from build123d import *
from build123d.topology import SkipClean

# Parameters (mm, degrees)
CUT_EXTRUDE1_DEPTH      = 35
CUT_EXTRUDE1_DEPTH_BACK = 35
SKETCH2_OUTSIDE_W       = 96.248
SKETCH2_OUTSIDE_H       = 96.248
BOSS_EXTRUDE1_DEPTH     = 46
SKETCH4_R               = 3.5
CUT_EXTRUDE2_DEPTH      = 5
LPATTERN1_COUNT         = 2
LPATTERN1_PITCH         = 35
SCALE1_SCALE            = 0.2286


with BuildPart() as part:
    # Sketch1 → Revolve2 (revolve)
    with BuildSketch(Plane(origin=(0, 0, 0), x_dir=(1, 0, 0), z_dir=(0, 1, 0))):
        with BuildLine():
            Line((0, 35), (0, -35))
            ThreePointArc((0, -35), (35, 0), (0, 35))
        make_face()
    revolve(axis=Axis((0, 0, -35), (0, 0, 1)))

    # Sketch2 outside → Cut-Extrude1 (cut, two sides: drawn at the far end of the back side and taken through both)
    with SkipClean():  # the faces are left unmerged after this step: merging them gives an invalid solid
        with BuildSketch(Plane(origin=(0, 0, 0), x_dir=(1, 0, 0), z_dir=(0, 1, 0)).offset(-CUT_EXTRUDE1_DEPTH_BACK)):
            Rectangle(SKETCH2_OUTSIDE_W, SKETCH2_OUTSIDE_H)
            with BuildLine():
                Line((-20, -28.722813233), (-20, 28.722813233))
                ThreePointArc((-20, 28.722813233), (0, 35), (20, 28.722813233))
                Line((20, 28.722813233), (20, -28.722813233))
                ThreePointArc((20, -28.722813233), (0, -35), (-20, -28.722813233))
            make_face(mode=Mode.SUBTRACT)
        extrude(amount=CUT_EXTRUDE1_DEPTH + CUT_EXTRUDE1_DEPTH_BACK, mode=Mode.SUBTRACT)

    # Sketch3 → Boss-Extrude1 (add)
    with BuildSketch(Plane(origin=(0, 0, 0), x_dir=(1, 0, 0), z_dir=(0, 1, 0))):
        with BuildLine():
            Line((-20, 15), (-20, -15))
            ThreePointArc((-20, -15), (0, -25), (20, -15))
            Line((20, -15), (20, 15))
            ThreePointArc((20, 15), (0, 25), (-20, 15))
        make_face()
    extrude(amount=BOSS_EXTRUDE1_DEPTH)

    # Sketch4 → Cut-Extrude2 (cut)
    with BuildSketch(Plane.ZY.offset(20)):
        Circle(SKETCH4_R)
    cut_extrude2 = extrude(amount=-CUT_EXTRUDE2_DEPTH, mode=Mode.SUBTRACT)

    # LPattern1: Cut-Extrude2 ×2
    with Locations(*[(i * LPATTERN1_PITCH, 0, 0) for i in range(1, LPATTERN1_COUNT)]):
        add(cut_extrude2, mode=Mode.SUBTRACT)


with BuildPart() as part_1:
    # Scale1: scaled about (-2.48e-07, 6.314524212, 6.409e-06)
    add(part.part.scale(SCALE1_SCALE).moved(Location((-1.91e-07, 4.871023977, 4.944e-06))))


solid = part_1.part
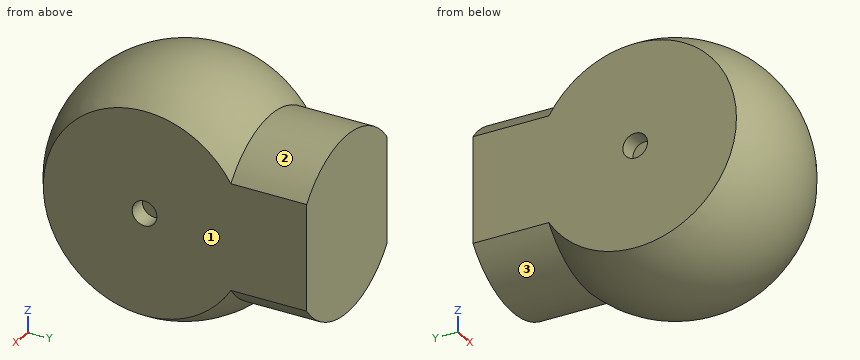
Geometry: final body of the model. Coordinates: model frame, mm. Face numbers are marked on the shaded views. A direction names the side the tool comes from. Give positions to 0.01 mm unless a question says otherwise; leave off trailing zeros. Loops run counter-clockwise (first coordinate to the right, second up) from the corner with the lowest first, then second, coordinate; pieces in that order, holes last. Notation, with made-up numbers: M 87.25,45.5 L 113.25,45.5 A20 cw 113.25,54.5 Z; hole C 8.25,75.25 d7. An arc over 180 degrees is marked long. Put each result on its own line as item: value.
1) Cut plane B-B, the plane z = 5.25. Return the cut outline in (x, y), plus the area to 3 significant figures.
Computed values:
outline: M -4.57,0.93 A6.04 ccw 4.57,0.93 L 4.57,8.81 A6.04 ccw 2.26,10.47 L 2.26,15.39 L -2.26,15.39 L -2.26,10.47 A6.04 ccw -4.57,8.81 Z
area: 120 mm^2
2) First-contact query: P1, Ø0.5, axis at y = 4.5, z = 0, coming from the -X side; P2, Ø3, axis at y = 12.5, z = 6, coming from the +X side; P3, Ø5, axis at x = 0, z = -4.5, coming from the -Y side. Flat tips, straight axial feed; report the tip coordinate or a pass-through.
Computed values:
P1: stops at x = -3.43
P2: stops at x = 3.52
P3: stops at y = -2.88
3) Reachability of the marked faces 1, 2 and 3 from +Z, -Z, +X, -X, +Y, -Y: full face, straight path, thin tool, end or side. Return the list, or none.
Computed values:
face 1: +Z, -Z, +X, +Y, -Y
face 2: +Z, +Y
face 3: -Z, +Y
4) Cut plane C-C, the plane y = 3.75. Return the cut outline in (x, z).
Computed values:
outline: M -4.57,-6.47 A7.92 ccw 4.57,-6.47 L 4.57,6.47 A7.92 ccw -4.57,6.47 Z
5) Material intervals for L1, parallel to Z at x = 2.75, y = 6.75; L2, parallel to Y at x = -3.5, z = -3.5; L3, parallel to Y at x = -1.75, z = -0.5, sorted ascending. Write a range as from..to.
Computed values:
L1: z = -7.27..7.27
L2: y = -1.42..15.39
L3: y = -2.92..15.39
6) Cut plane A-A, the plane x = -4. Return the cut outline in (y, z), plus the area to 3 significant figures.
Computed values:
outline: M 10.47,-4.08 L 15.39,-4.08 L 15.39,4.08 L 10.47,4.08 A6.93 ccw long Z; hole C 4.87,0 d1.6
area: 182 mm^2
7) Cut plane D-D, the plane x = -1.75. Return the cut outline in (y, z).
Computed values:
outline: M 10.47,-5.44 L 15.39,-5.44 L 15.39,5.44 L 10.47,5.44 A7.81 ccw long Z
